from build123d import *

# Parameters (mm, degrees)
F0_W        = 29
F0_H        = 14
F0_W_2      = 25
F0_H_2      = 10
F1_DEPTH    = 20
F2_W        = 15
F2_H        = 2
F3_DEPTH    = 15
F5_DEPTH    = 2
F6_T1_DEPTH = 2
F6_T3_DEPTH = 2
F6_T5_DEPTH = 39.5
F6_T7_DEPTH = 39.5


# Not quite as in the source:
# - a fillet or chamfer that OpenCascade refuses, or shapes differently, is made with other operations: its cross-section is extruded or revolved along the edge and cut away or added


with BuildPart() as f1:
    # F0 (on Top) → F1 (new body)
    with BuildSketch(Plane.XY):
        with Locations((14.5, -7)):
            Rectangle(F0_W, F0_H)
        with Locations((14.5, -7)):
            Rectangle(F0_W_2, F0_H_2, mode=Mode.SUBTRACT)
    extrude(amount=F1_DEPTH)

    # F2 (on face) → F3 (join)
    with BuildSketch(Plane.XY.offset(20)):
        with Locations((14.5, -1)):
            Rectangle(F2_W, F2_H)
    extrude(amount=F3_DEPTH)

    # F4 (on face) → F5 (cut, through all)
    with BuildSketch(Plane.XZ.offset(2)):
        with BuildLine():
            Line((17.8888604279, 25.875), (16.4364916731, 31.5))
            ThreePointArc((16.4364916731, 31.5), (14.5, 33), (12.5635083269, 31.5))
            Line((12.5635083269, 31.5), (11.1111395721, 25.875))
            ThreePointArc((11.1111395721, 25.875), (14.5, 21.5), (17.8888604279, 25.875))
        make_face()
    extrude(amount=-F5_DEPTH, mode=Mode.SUBTRACT)

    # F6: fillet of radius 7.5 on 4 edges, made by hand

    # F6_s2 → F6_t1 (join)
    with BuildSketch(Plane.XZ):
        with BuildLine():
            ThreePointArc((0, 20), (4.9772255751, 22.3598393906), (7, 27.4833147735))
            Line((7, 27.4833147735), (7, 20))
            Line((7, 20), (0, 20))
        make_face()
    extrude(amount=F6_T1_DEPTH)

    # F6_s4 → F6_t3 (join)
    with BuildSketch(Plane.XZ):
        with BuildLine():
            ThreePointArc((29, 20), (24.0227744249, 22.3598393906), (22, 27.4833147735))
            Line((22, 27.4833147735), (22, 20))
            Line((22, 20), (29, 20))
        make_face()
    extrude(amount=F6_T3_DEPTH)

    # F6_s6 → F6_t5 (cut)
    with BuildSketch(Plane.XZ.offset(-18.75)):
        with BuildLine():
            ThreePointArc((22, 27.5), (19.8033008589, 32.8033008589), (14.5, 35))
            Line((14.5, 35), (22, 35))
            Line((22, 35), (22, 27.5))
        make_face()
    extrude(amount=F6_T5_DEPTH, mode=Mode.SUBTRACT)

    # F6_s8 → F6_t7 (cut)
    with BuildSketch(Plane.XZ.offset(-18.75)):
        with BuildLine():
            ThreePointArc((7, 27.5), (9.1966991411, 32.8033008589), (14.5, 35))
            Line((14.5, 35), (7, 35))
            Line((7, 35), (7, 27.5))
        make_face()
    extrude(amount=F6_T7_DEPTH, mode=Mode.SUBTRACT)


solid = f1.part
Could you check a few things on this model? Use its own coordinates, in mm. A direction names the side the tool comes from. Round coordinates to 2 decimals unless told otherwise and drop trailing zeros. Order: outer loops, then holes, each group sorted by start corner. A loop starts at its lowest first (then second) coordinate and runs counter-clockwise, first axis right, second up.
(1) Imagine slicing it at C-C (z = 31). Write out the boundary of the cut face in (x, y), plus the area to 3 significant figures.
Response values:
outline: (7.87, -2) - (12.43, -2) - (12.43, 0) - (7.87, 0) - close; (16.57, -2) - (21.13, -2) - (21.13, 0) - (16.57, 0) - close
area: 18.3 mm2
(2) I'm going to push flat-ended pins straight in: pin 1 (3 mm diameter, centred on x = 14.5, y = -4, fed in from -Z); pin 2 (8 mm diameter, centred on x = 8, z = 26.5, fed in from -Y). Where does each tip first touch, or does it pass through?
Response values:
pin 1: passes through
pin 2: stops at y = -2
(3) Imagine slicing it at D-D (y = -8.5). Write out the boundary of the cut face in (x, z), plus the area to 3 significant figures.
Response values:
outline: (0, 0) - (2, 0) - (2, 20) - (0, 20) - close; (27, 0) - (29, 0) - (29, 20) - (27, 20) - close
area: 80.0 mm2
(4) Which directions (+Z, -Z, +X, -X, +Y, -Y) give clear straight access to the entire face, cutting with the end or side of a thin tool? Please do faces 1 (the flat face through (15.5, -12.4, 20)), 2 (the flat face through (2, -7, 10)), 3 (the cylindrical face through (14.5, -1, 33)).
Response values:
face 1: +Z, +X, -X, -Y
face 2: +Z, -Z
face 3: +Y, -Y
(5) Imagine slicing it at A-A (x = 14.5). Write out the boundary of the cut face in (y, z).
Response values:
outline: (-14, 0) - (-12, 0) - (-12, 20) - (-14, 20) - close; (-2, 0) - (0, 0) - (0, 21.5) - (-2, 21.5) - close; (-2, 33) - (0, 33) - (0, 35) - (-2, 35) - close
(6) If we mould it in two halves opening along X, with no side actions, what happens to faces 4 (the flat face through (29, -7, 10)), 5 (the cylindrical face through (14.4, -1, 21.5)), 6 (the flat face through (14, 0, 14))? For each: released by +X, released by -X, zero draft, split by the parting line, or undercut.
Response values:
face 4: released by +X
face 5: undercut
face 6: zero draft
(7) Please list where these lines run through material, in increasing order: line 1 along Y through (x, z) = (12.5, 18); line 2 along X through (y, z) = (-7.5, 3); line 3 along Y through (x, z) = (9.25, 28.5).
Response values:
line 1: y = -14 to -12, -2 to 0
line 2: x = 0 to 2, 27 to 29
line 3: y = -2 to 0
